Design review of the part built by this model. Coordinates are the model's own, in mm. Face numbers are marked on the shaded views. A direction names the side the tool comes from. Round coordinates to 2 decimals unless told otherwise and drop trailing zeros. Order: outer loops, then holes, each group sorted by start corner. A loop starts at its lowest first (then second) coordinate and runs counter-clockwise, first axis right, second up. Notation, with made-up numbers: (41.5, 17) - (78.5, 17) arc R30 ccw to (78.5, 41) - close; hole circle Ø2 at (18, 80). An arc over 180 degrees is marked (long way). Write item = value, one per line.
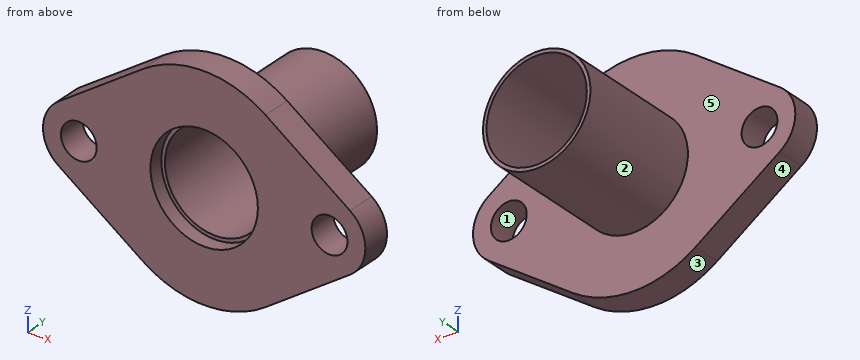
from build123d import *

# Parameters (mm, degrees)
F0_R     = 3.175
F0_R_2   = 9.525
F1_DEPTH = 2.54
F2_DEPTH = 25.4
F3_D     = 17.78


with BuildPart() as f1:
    # F0 (on Front) → F1 (new body, symmetric)
    with BuildSketch(Plane.XZ):
        with BuildLine():
            Line((-25.8535714286, -5.2111389722), (-10.8857142857, -15.6334169166))
            ThreePointArc((-10.8857142857, -15.6334169166), (0, -19.05), (10.8857142857, -15.6334169166))
            Line((10.8857142857, -15.6334169166), (25.8535714286, -5.2111389722))
            ThreePointArc((25.8535714286, -5.2111389722), (28.575, 0), (25.8535714286, 5.2111389722))
            Line((25.8535714286, 5.2111389722), (10.8857142857, 15.6334169166))
            ThreePointArc((10.8857142857, 15.6334169166), (0, 19.05), (-10.8857142857, 15.6334169166))
            Line((-10.8857142857, 15.6334169166), (-25.8535714286, 5.2111389722))
            ThreePointArc((-25.8535714286, 5.2111389722), (-28.575, 0), (-25.8535714286, -5.2111389722))
        make_face()
        with Locations((-22.225, 0)):
            Circle(F0_R, mode=Mode.SUBTRACT)
        Circle(F0_R_2, mode=Mode.SUBTRACT)
        with Locations((22.225, 0)):
            Circle(F0_R, mode=Mode.SUBTRACT)
    extrude(amount=F1_DEPTH, both=True)

    # F0 (on Front) → F2 (join)
    with BuildSketch(Plane.XZ):
        Circle(F0_R_2)
    extrude(amount=-F2_DEPTH)

    # F3 (through all)
    with Locations(Plane.XZ):
        with Locations((0, 0)):
            Hole(F3_D / 2)


solid = f1.part
Item 1: For line 1 along Z through (x, y) = (0, -0.55) (3 decimals); line 2 along Z through (x, y) = (0, 24.25) (3 decimals); line 3 along Y through (x, z) = (6.5, -6.5), list the stretches that pass through material, from the lowest coordinate up. Write a range as [from, to].
Data:
line_1 = [-19.05, -9.525], [9.525, 19.05]
line_2 = [-9.525, -8.89], [8.89, 9.525]
line_3 = [0, 25.4]
Item 2: Take a section at D-D, the plane y = 16.5. State the section outline as (x, z) points (3 decimals), and give its area (3 significant figures).
Data:
outline = circle Ø19.05 at (0, 0); hole circle Ø17.78 at (0, 0)
area = 36.7 mm2
Item 3: The part is to be moulded in two halves that separate along Z. For the marked faces 1, 2 and 3, say which applies: +Z half, -Z half, draft (parallel to the pull), parting line (faces both ways), or undercut.
Data:
face_1 = undercut
face_2 = parting line
face_3 = -Z half
Item 4: For the marked faces 4 and 5, list the 3-axis set-ups (+Z, -Z, +X, -X, +Y, -Y) from which the entire face can be reached by the end or side of a thin tool; tool diameter is ignored.
Data:
face_4 = -Z, -X, +Y, -Y
face_5 = +Y
Item 5: Take a section at C-C, the plane z = -6. State the section outline as (x, y) points.
Data:
outline = (-24.72, -2.54) - (-7.4, -2.54) - (-7.4, 0) - (-6.56, 0) - (-6.56, 25.4) - (-7.4, 25.4) - (-7.4, 2.54) - (-24.72, 2.54) - close; (6.56, 0) - (7.4, 0) - (7.4, -2.54) - (24.72, -2.54) - (24.72, 2.54) - (7.4, 2.54) - (7.4, 25.4) - (6.56, 25.4) - close
Item 6: Insertion check: P1, Ø10, axis at y = 1.5, z = 15, coming from the +X side; P2, Ø6, axis at y = 2.5, z = -10, coming from the -X side; P3, Ø4, axis at x = -8, y = 15.5, coming from the -Z side. Each pin has a flat end and moves straight along its axis. Give the tip position at first contact, or say it passes through.
Data:
P1 = 18.98
P2 = -23.28
P3 = -7.4
Item 7: Take a section at B-B, the plane z = 0. State the section outline as (x, y) points (3 decimals).
Data:
outline = (-28.575, -2.54) - (-25.4, -2.54) - (-25.4, 2.54) - (-28.575, 2.54) - close; (-19.05, -2.54) - (-9.525, -2.54) - (-9.525, 0) - (-8.89, 0) - (-8.89, 25.4) - (-9.525, 25.4) - (-9.525, 2.54) - (-19.05, 2.54) - close; (8.89, 0) - (9.525, 0) - (9.525, -2.54) - (19.05, -2.54) - (19.05, 2.54) - (9.525, 2.54) - (9.525, 25.4) - (8.89, 25.4) - close; (25.4, -2.54) - (28.575, -2.54) - (28.575, 2.54) - (25.4, 2.54) - close
Item 8: Take a section at A-A, the plane x = 0. State the section outline as (y, z) points (3 decimals).
Data:
outline = (-2.54, -19.05) - (2.54, -19.05) - (2.54, -9.525) - (25.4, -9.525) - (25.4, -8.89) - (0, -8.89) - (0, -9.525) - (-2.54, -9.525) - close; (-2.54, 9.525) - (0, 9.525) - (0, 8.89) - (25.4, 8.89) - (25.4, 9.525) - (2.54, 9.525) - (2.54, 19.05) - (-2.54, 19.05) - close
